Answer from the drawing. Dimensions are ordinates in mm from the lowest x, y and z of the part. Round coordinates to 2 decimals unless told otherwise and drop trailing zeros. Write each loop counter-clockwise with the first axis right and the second up, starting at its lowest first coordinate (ties: lowest second). Pieces come first, ordered by that corner, then holes. Notation, with made-up numbers: (45.5, 8) - (51.5, 8) arc R16 ccw to (51.5, 22) - close; hole circle Ø10 at (47, 35.25). An arc over 180 degrees is marked (long way). Answer as CSV lines item,"result". Start each with the question number.
1) Each of these flat-tipped pins is pushed along its axis until it touches: pin 1 (0.6 mm diameter, centred on x = 1, z = 5.5, fed in from -Y); pin 2 (0.8 mm diameter, centred on x = 2, y = 20.5, fed in from -Z); pin 3 (1.5 mm diameter, centred on y = 33.5, z = 1, fed in from +X); pin 4 (1.2 mm diameter, centred on y = 5.38, z = 3.09, fed in from +X). Where does it stop, or does it pass through?
2) Find section B-B on z = 2.5. Determine the outline of the cut face in (x, y).
3) Consider line 1 along Y through (x, z) = (1, 3); line 2 along Z through (x, y) = (0.3, 3.5); line 3 along X through (y, z) = (5, 0.5). Determine where each line is inside the solid, lowest interval first.
4) Find section D-D on z = 5.5. Determine the outline of the cut face in (x, y).
5) Find section A-A on x = 0.75. State how many separate pieces and enclosed holes the cut face has.
6) Find section C-C on y = 8.5. Determine the outline of the cut face in (x, z).
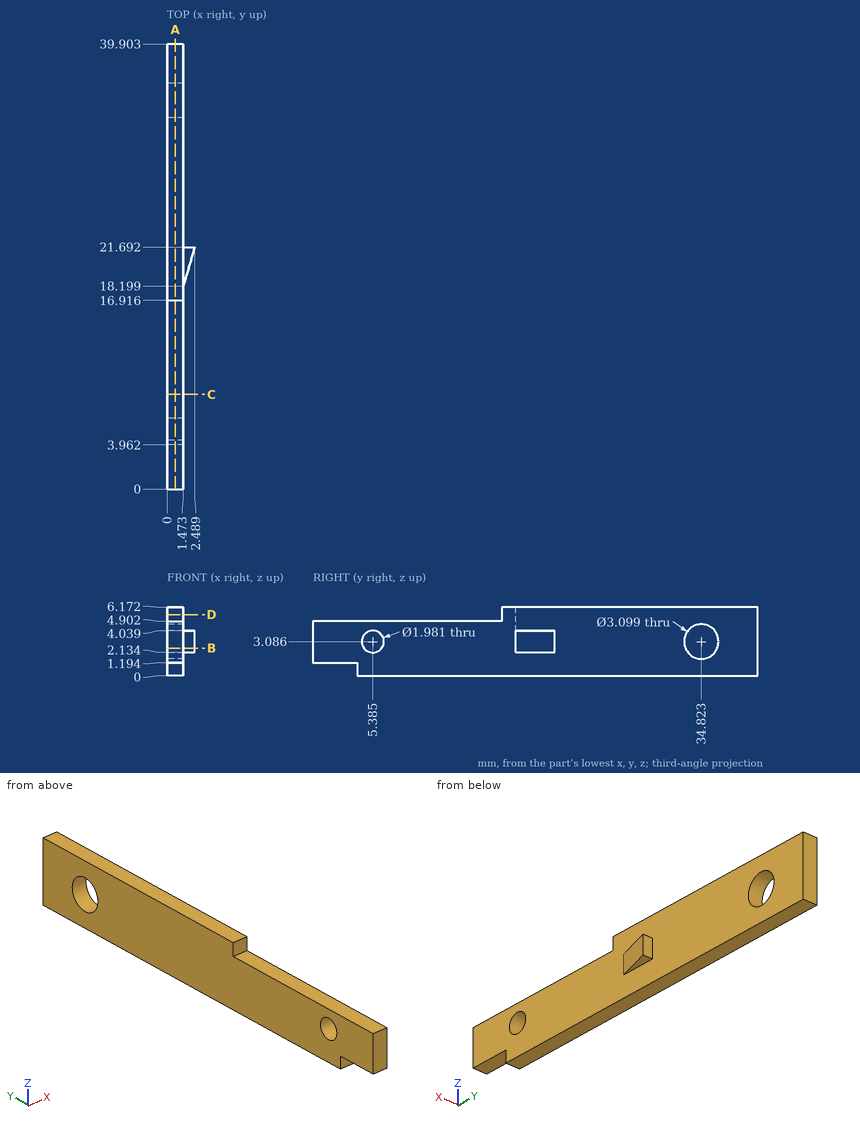
Check values:
1,pin 1,"stops at y = 16.92"
1,pin 2,"stops at z = 2.13"
1,pin 3,"stops at x = 1.47"
1,pin 4,"passes through"
2,outline,"(0, 0) - (1.47, 0) - (1.47, 4.59) - (0, 4.59) - close; (0, 6.18) - (1.47, 6.18) - (1.47, 18.2) - (2.49, 21.69) - (1.47, 21.69) - (1.47, 33.39) - (0, 33.39) - close; (0, 36.26) - (1.47, 36.26) - (1.47, 39.9) - (0, 39.9) - close"
3,line 1,"y = 0 to 4.4, 6.37 to 33.28, 36.37 to 39.9"
3,line 2,"z = 1.19 to 4.9"
3,line 3,"x = 0 to 1.47"
4,outline,"(0, 16.92) - (1.47, 16.92) - (1.47, 39.9) - (0, 39.9) - close"
5,separate pieces,"1"
5,enclosed holes,"2"
6,outline,"(0, 0) - (1.47, 0) - (1.47, 4.9) - (0, 4.9) - close"
